Autodesk Inventor part; units mm, degrees
ref_plane "YZ Plane" through (0, 0, 0) normal (1, 0, 0) x (0, 1, 0)
ref_plane "XZ Plane" through (0, 0, 0) normal (0, 1, 0) x (-1, 0, 0)
ref_plane "XY Plane" through (0, 0, 0) normal (0, 0, 1) x (1, 0, 0)
sketch "Skizze1" plane through (0, 0, 0) normal (0, 0, 1) x (1, 0, 0)
  arc A0 (6, 0) -> (-6, 0) centre (0, 0) ccw
  arc A1 (7.5, 0) -> (-7.5, 0) centre (0, 0) ccw
  arc A2 (-6, -305.0274) -> (6, -305.0274) centre (0, -305.0274) ccw
  line L0 (0, -305.0274) -> (6, -305.0274) construction
  line L1 (0, -305.0274) -> (-6, -305.0274) construction
  arc A3 (-7.5, -305.0274) -> (7.5, -305.0274) centre (0, -305.0274) ccw
  line L2 (0, -305.0274) -> (7.5, -305.0274) construction
  line L3 (0, -305.0274) -> (-7.5, -305.0274) construction
  line L4 (-7.5, -305.0274) -> (-7.5, 0)
  line L5 (-6, 0) -> (-6, -305.0274)
  line L6 (6, -305.0274) -> (6, 0)
  line L7 (7.5, -305.0274) -> (7.5, 0)
  dimension "d0" = 6
  dimension "d1" = 7.5
  dimension "d2" = 6
  dimension "d3" = 180
  dimension "d4" = 7.5
  dimension "d5" = 180
  dimension "d6" = 305.0274
  dimension "d7" = 0
extrude "Extrusion1" add sketch "Skizze1" along normal blind 6
properties part number "Y belt" material "Gummi, Silikon"
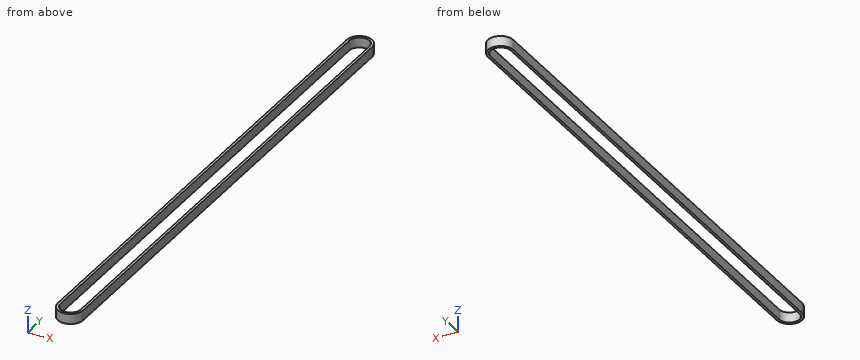
Can you work these out from the model? Positions are in its coordinate system, mm. Give positions to 0.01 mm unless a question says otherwise; leave off trailing zeros. Loops run counter-clockwise (first coordinate to the right, second up) from the corner with the lowest first, then second, coordinate; pieces in that order, holes last. Notation, with made-up numbers: (-3.5, 5.5) -> (36.5, 5.5) arc R33 cw to (36.5, 34.5) -> close; hole circle Ø5 at (-23.5, 0.25). An arc over 180 degrees is marked (long way). Write item = value, one per line.
1) Suppose I cut it at B-B on z = 4.2. Write out the boundary of the cut face in (x, y), then the cut area to 3 significant figures.
Check result:
outline = (-7.5, -305.03) arc R7.5 ccw to (7.5, -305.03) -> (7.5, 0) arc R7.5 ccw to (-7.5, 0) -> close; hole (-6, -305.03) arc R6 ccw to (6, -305.03) -> (6, 0) arc R6 ccw to (-6, 0) -> close
area = 979 mm2
2) Suppose I cut it at A-A on y = -251.5. Write out the boundary of the cut face in (x, z).
Check result:
outline = (-7.5, 0) -> (-6, 0) -> (-6, 6) -> (-7.5, 6) -> close; (6, 0) -> (7.5, 0) -> (7.5, 6) -> (6, 6) -> close
3) Will these pins go through, and if not, where does the flat tip stop? pin 1 (1 mm diameter, centred on x = 6, y = -63.5, fed in from -Z); pin 2 (2 mm diameter, centred on x = -3.5, y = -62.5, fed in from +Z); pin 3 (1 mm diameter, centred on x = -1.5, z = 5, fed in from -Y).
Check result:
pin_1 = 0
pin_2 = through
pin_3 = -312.46
4) I need wall thicknesses on L1, parallel to X at y = -63.5, z = 4.6; L2, parallel to Y at x = 0.75, z = 4.55; L3, parallel to Y at x = 2.5, z = 5. Which ranges of each line are inside material? Lowest first, please. Write a range as from..to.
Check result:
L1 = -7.5..-6, 6..7.5
L2 = -312.49..-310.98, 5.95..7.46
L3 = -312.1..-310.48, 5.45..7.07
5) Suppose I cut it at C-C on x = 0. Write out the boundary of the cut face in (y, z), then the cut area to 3 significant figures.
Check result:
outline = (-312.53, 0) -> (-311.03, 0) -> (-311.03, 6) -> (-312.53, 6) -> close; (6, 0) -> (7.5, 0) -> (7.5, 6) -> (6, 6) -> close
area = 18.0 mm2
